from build123d import *

# Parameters (mm, degrees)
SKETCH_1_W                      = 158
SKETCH_1_H                      = 47.848101266
EXTRUDE_1_DEPTH                 = 2.5
CUT_EXTRUDE_1_REACH             = 84.581
SKETCH_2_W                      = 64
SKETCH_2_H                      = 27.924050633
CUT_EXTRUDE_2_REACH             = 84.581
SKETCH_4_R                      = 1.7
SKETCH_4_R_2                    = 1.8
CUT_EXTRUDE_3_REACH             = 84.581
SKETCH_5_R                      = 1.6
CUT_EXTRUDE_3_DIRECTION_2_DEPTH = 83.580931205
FILLET_4_R                      = 3
FILLET_5_R                      = 4
FILLET_6_R                      = 20
EXTRUDE_START                   = -79
EXTRUDE_2_DEPTH                 = 65
CUT_EXTRUDE_START               = -79
CUT_EXTRUDE_4_DEPTH             = 40
FILLET_7_R                      = 0.5
FILLET_8_R                      = 2
FILLET_9_R                      = 3
FILLET_10_R                     = 2
SKETCH_10_R                     = 1.6
CUT_EXTRUDE_5_DEPTH             = 95.325235224
SKETCH_11_R                     = 1.6
CUT_EXTRUDE_6_DEPTH             = 85.602511087


with BuildPart() as part:
    # 草图1 → 凸台-拉伸1 (new body)
    with BuildSketch(Plane(origin=(0, 0, 0), x_dir=(1, 0, 0), z_dir=(0, 1, 0))):
        Rectangle(SKETCH_1_W, SKETCH_1_H)
    extrude(amount=EXTRUDE_1_DEPTH)

    # 草图2 → 切除-拉伸1 (cut, up to next)
    with BuildSketch(Plane(origin=(0, 2.5, 0), x_dir=(1, 0, 0), z_dir=(0, 1, 0)), mode=Mode.PRIVATE) as cut_extrude_1_sk1:
        with Locations((-32, -9.962025317)):
            Rectangle(SKETCH_2_W, SKETCH_2_H)
    cut_extrude_1_tool1 = extrude(cut_extrude_1_sk1.sketch, amount=-CUT_EXTRUDE_1_REACH, mode=Mode.PRIVATE) & part.part
    # 草图2 → 切除-拉伸1 (cut, up to next)
    with BuildSketch(Plane(origin=(0, 2.5, 0), x_dir=(1, 0, 0), z_dir=(0, 1, 0)), mode=Mode.PRIVATE) as cut_extrude_1_sk2:
        with Locations((32, -9.962025317)):
            Rectangle(SKETCH_2_W, SKETCH_2_H)
    cut_extrude_1_tool2 = extrude(cut_extrude_1_sk2.sketch, amount=-CUT_EXTRUDE_1_REACH, mode=Mode.PRIVATE) & part.part
    add(cut_extrude_1_tool1.solids().sort_by_distance((-32, 2.5, 9.962025))[0], mode=Mode.SUBTRACT)
    add(cut_extrude_1_tool2.solids().sort_by_distance((32, 2.5, 9.962025))[0], mode=Mode.SUBTRACT)

    # 草图4 → 切除-拉伸2 (cut, up to next)
    with BuildSketch(Plane(origin=(0, 2.5, 0), x_dir=(1, 0, 0), z_dir=(0, 1, 0)), mode=Mode.PRIVATE) as cut_extrude_2_sk1:
        with Locations(Location((-74, -8.924050633, 0), (0, 0, 270))):
            Circle(SKETCH_4_R)
    cut_extrude_2_tool1 = extrude(cut_extrude_2_sk1.sketch, amount=-CUT_EXTRUDE_2_REACH, mode=Mode.PRIVATE) & part.part
    # 草图4 → 切除-拉伸2 (cut, up to next)
    with BuildSketch(Plane(origin=(0, 2.5, 0), x_dir=(1, 0, 0), z_dir=(0, 1, 0)), mode=Mode.PRIVATE) as cut_extrude_2_sk2:
        with Locations(Location((-74, 20.575949367, 0), (0, 0, 270))):
            Circle(SKETCH_4_R)
    cut_extrude_2_tool2 = extrude(cut_extrude_2_sk2.sketch, amount=-CUT_EXTRUDE_2_REACH, mode=Mode.PRIVATE) & part.part
    # 草图4 → 切除-拉伸2 (cut, up to next)
    with BuildSketch(Plane(origin=(0, 2.5, 0), x_dir=(1, 0, 0), z_dir=(0, 1, 0)), mode=Mode.PRIVATE) as cut_extrude_2_sk3:
        with Locations(Location((-74, -19.424050633, 0), (0, 0, 270))):
            Circle(SKETCH_4_R_2)
    cut_extrude_2_tool3 = extrude(cut_extrude_2_sk3.sketch, amount=-CUT_EXTRUDE_2_REACH, mode=Mode.PRIVATE) & part.part
    # 草图4 → 切除-拉伸2 (cut, up to next)
    with BuildSketch(Plane(origin=(0, 2.5, 0), x_dir=(1, 0, 0), z_dir=(0, 1, 0)), mode=Mode.PRIVATE) as cut_extrude_2_sk4:
        with Locations(Location((74, 20.575949367, 0), (0, 0, 270))):
            Circle(SKETCH_4_R)
    cut_extrude_2_tool4 = extrude(cut_extrude_2_sk4.sketch, amount=-CUT_EXTRUDE_2_REACH, mode=Mode.PRIVATE) & part.part
    # 草图4 → 切除-拉伸2 (cut, up to next)
    with BuildSketch(Plane(origin=(0, 2.5, 0), x_dir=(1, 0, 0), z_dir=(0, 1, 0)), mode=Mode.PRIVATE) as cut_extrude_2_sk5:
        with Locations(Location((74, -19.424050633, 0), (0, 0, 270))):
            Circle(SKETCH_4_R_2)
    cut_extrude_2_tool5 = extrude(cut_extrude_2_sk5.sketch, amount=-CUT_EXTRUDE_2_REACH, mode=Mode.PRIVATE) & part.part
    # 草图4 → 切除-拉伸2 (cut, up to next)
    with BuildSketch(Plane(origin=(0, 2.5, 0), x_dir=(1, 0, 0), z_dir=(0, 1, 0)), mode=Mode.PRIVATE) as cut_extrude_2_sk6:
        with Locations(Location((74, -8.924050633, 0), (0, 0, 270))):
            Circle(SKETCH_4_R)
    cut_extrude_2_tool6 = extrude(cut_extrude_2_sk6.sketch, amount=-CUT_EXTRUDE_2_REACH, mode=Mode.PRIVATE) & part.part
    add(cut_extrude_2_tool1.solids().sort_by_distance((-74, 2.5, 8.924051))[0], mode=Mode.SUBTRACT)
    add(cut_extrude_2_tool2.solids().sort_by_distance((-74, 2.5, -20.575949))[0], mode=Mode.SUBTRACT)
    add(cut_extrude_2_tool3.solids().sort_by_distance((-74, 2.5, 19.424051))[0], mode=Mode.SUBTRACT)
    add(cut_extrude_2_tool4.solids().sort_by_distance((74, 2.5, -20.575949))[0], mode=Mode.SUBTRACT)
    add(cut_extrude_2_tool5.solids().sort_by_distance((74, 2.5, 19.424051))[0], mode=Mode.SUBTRACT)
    add(cut_extrude_2_tool6.solids().sort_by_distance((74, 2.5, 8.924051))[0], mode=Mode.SUBTRACT)

    # 草图5 → 切除-拉伸3 (cut, up to next)
    with BuildSketch(Plane(origin=(0, 2.5, 0), x_dir=(1, 0, 0), z_dir=(0, 1, 0)), mode=Mode.PRIVATE) as cut_extrude_3_sk1:
        with Locations(Location((0, 14, 0), (0, 0, 90))):
            Circle(SKETCH_5_R)
    cut_extrude_3_tool1 = extrude(cut_extrude_3_sk1.sketch, amount=-CUT_EXTRUDE_3_REACH, mode=Mode.PRIVATE) & part.part
    # 草图5 → 切除-拉伸3 (cut, up to next)
    with BuildSketch(Plane(origin=(0, 2.5, 0), x_dir=(1, 0, 0), z_dir=(0, 1, 0)), mode=Mode.PRIVATE) as cut_extrude_3_sk2:
        with Locations(Location((-45, 14, 0), (0, 0, 90))):
            Circle(SKETCH_5_R)
    cut_extrude_3_tool2 = extrude(cut_extrude_3_sk2.sketch, amount=-CUT_EXTRUDE_3_REACH, mode=Mode.PRIVATE) & part.part
    # 草图5 → 切除-拉伸3 (cut, up to next)
    with BuildSketch(Plane(origin=(0, 2.5, 0), x_dir=(1, 0, 0), z_dir=(0, 1, 0)), mode=Mode.PRIVATE) as cut_extrude_3_sk3:
        with Locations(Location((45, 14, 0), (0, 0, 90))):
            Circle(SKETCH_5_R)
    cut_extrude_3_tool3 = extrude(cut_extrude_3_sk3.sketch, amount=-CUT_EXTRUDE_3_REACH, mode=Mode.PRIVATE) & part.part
    add(cut_extrude_3_tool1.solids().sort_by_distance((0, 2.5, -14))[0], mode=Mode.SUBTRACT)
    add(cut_extrude_3_tool2.solids().sort_by_distance((-45, 2.5, -14))[0], mode=Mode.SUBTRACT)
    add(cut_extrude_3_tool3.solids().sort_by_distance((45, 2.5, -14))[0], mode=Mode.SUBTRACT)

    # 草图5 → 切除-拉伸3 direction 2 (cut)
    with BuildSketch(Plane(origin=(0, 2.5, 0), x_dir=(1, 0, 0), z_dir=(0, 1, 0))):
        with Locations(Location((0, 14, 0), (0, 0, 90))):
            Circle(SKETCH_5_R)
        with Locations(Location((-45, 14, 0), (0, 0, 90))):
            Circle(SKETCH_5_R)
        with Locations(Location((45, 14, 0), (0, 0, 90))):
            Circle(SKETCH_5_R)
    extrude(amount=CUT_EXTRUDE_3_DIRECTION_2_DEPTH, mode=Mode.SUBTRACT)

    # 圆角4
    fillet_4_edges = [part.edges().sort_by_distance(p)[0] for p in [
        (79, 1.25, 23.924050633),
        (-79, 1.25, 23.924050633),
        (-79, 1.25, -23.924050633),
        (79, 1.25, -23.924050633),
    ]]
    fillet(fillet_4_edges, radius=FILLET_4_R)

    # 圆角5
    fillet_5_edges = [part.edges().sort_by_distance(p)[0] for p in [
        (64, 1.25, 23.924050633),
        (-64, 1.25, 23.924050633),
    ]]
    fillet(fillet_5_edges, radius=FILLET_5_R)

    # 圆角6
    fillet_6_edges = [part.edges().sort_by_distance(p)[0] for p in [
        (-64, 1.25, -4),
        (64, 1.25, -4),
    ]]
    fillet(fillet_6_edges, radius=FILLET_6_R)

    # 草图8 → 凸台-拉伸2 (add, symmetric)
    with BuildSketch(Plane.ZY.offset(79).offset(EXTRUDE_START)):
        Polygon((-22.743286719, 0), (-28.575949367, 0), (-28.575949367, 12.5), (-26.075949367, 12.5), (-26.075949367, 2.5), (-22.743286719, 2.5), align=None)
    extrude(amount=EXTRUDE_2_DEPTH, both=True)

    # 草图9 → 切除-拉伸4 (cut, symmetric)
    with BuildSketch(Plane.ZY.offset(79).offset(CUT_EXTRUDE_START)):
        Polygon((-28.575949367, 0), (-22.743286719, 0), (-22.743286719, 2.5), (-26.075949367, 2.5), (-26.075949367, 12.5), (-28.575949367, 12.5), align=None)
    extrude(amount=CUT_EXTRUDE_4_DEPTH, both=True, mode=Mode.SUBTRACT)

    # 圆角7
    fillet_7_edges = [part.edges().sort_by_distance(p)[0] for p in [
        (52.5, 2.5, -26.075949367),
        (-52.5, 2.5, -26.075949367),
    ]]
    fillet(fillet_7_edges, radius=FILLET_7_R)

    # 圆角8
    fillet_8_edges = [part.edges().sort_by_distance(p)[0] for p in [
        (52.5, 0, -28.575949367),
        (-52.5, 0, -28.575949367),
    ]]
    fillet(fillet_8_edges, radius=FILLET_8_R)

    # 圆角9
    fillet_9_edges = [part.edges().sort_by_distance(p)[0] for p in [
        (-65, 12.5, -27.325949367),
        (65, 12.5, -27.325949367),
        (40, 12.5, -27.325949367),
        (-40, 12.5, -27.325949367),
    ]]
    fillet(fillet_9_edges, radius=FILLET_9_R)

    # 圆角10
    fillet_10_edges = [part.edges().sort_by_distance(p)[0] for p in [
        (-65, 1.25, -23.924050633),
        (-40, 1.25, -22.743286719),
        (65, 1.25, -23.924050633),
        (40, 1.25, -22.743286719),
    ]]
    fillet(fillet_10_edges, radius=FILLET_10_R)

    # 草图10 → 切除-拉伸5 (cut, through all)
    with BuildSketch(Plane.XY.offset(-26.075949367)):
        with Locations((-57.5, 7.5)):
            Circle(SKETCH_10_R)
        with Locations((-47.5, 7.5)):
            Circle(SKETCH_10_R)
        with Locations(Location((47.5, 7.5, 0), (0, 0, 180))):
            Circle(SKETCH_10_R)
        with Locations(Location((57.5, 7.5, 0), (0, 0, 180))):
            Circle(SKETCH_10_R)
    extrude(amount=-CUT_EXTRUDE_5_DEPTH, mode=Mode.SUBTRACT)

    # 草图11 → 切除-拉伸6 (cut, through all)
    with BuildSketch(Plane(origin=(0, 2.5, 0), x_dir=(1, 0, 0), z_dir=(0, 1, 0))):
        with Locations(Location((-27, 14, 0), (0, 0, 270))):
            Circle(SKETCH_11_R)
        with Locations(Location((-21, 14, 0), (0, 0, 270))):
            Circle(SKETCH_11_R)
        with Locations(Location((21, 14, 0), (0, 0, 90))):
            Circle(SKETCH_11_R)
        with Locations(Location((27, 14, 0), (0, 0, 90))):
            Circle(SKETCH_11_R)
    extrude(amount=-CUT_EXTRUDE_6_DEPTH, mode=Mode.SUBTRACT)


solid = part.part
Verification items for the finished model (mm, model axes). A direction names the side the tool comes from. Coordinates: 2 decimals unless noted, no trailing zeros. Order: outer loops, then holes, each group sorted by start corner. A loop starts at its lowest first (then second) coordinate and runs counter-clockwise, first axis right, second up. Notation, with made-up numbers: M -17,82.5 L 7,82.5 A22 ccw 7,105.5 Z; hole C -31,46 d2. An arc over 180 degrees is marked long. One line per item, written item: value. Start each with the question number.
Item 1: Sectioned sample at A-A (x = 0). Enter the section's corners in (y, z), then the cut area to 3 significant figures.
Item 2: Sectioned sample at D-D (z = -8.5). Enter the section's corners in (x, y).
Item 3: Sectioned sample at C-C (x = -18). Enter the section's corners in (y, z), then the cut area to 3 significant figures.
Item 4: Sectioned sample at B-B (y = 11). Enter the section's corners in (x, z), then the cut area to 3 significant figures.
Item 5: Access from +Z, -Z, +X, -X, +Y, -Y to the whole of each face (thin tool, end or side, straight path). Record for faces 1 (the cylindrical face through (65.14, 1.23, 22.72)), 2 (the flat face through (65, 5, -27)), 3 (the flat face through (-1, 2.5, -7)).
Item 6: Mould release check, pull along Y, two halves, no side actions. Record for faces 4 (the cylindrical face through (64.14, 11.6, -27.31)), 5 (the cylindrical face through (-56.02, 6.89, -27.31)), 6 (the cylindrical face through (-19.92, 1.27, -15.18)): released by +Y, released by -Y, zero draft, split by the parting line, or undercut.
Item 7: Scan lines: probe 1 along Z at (x, y) = (-74, 1.3); probe 2 along Y at (x, z) = (-51, -23.5); probe 3 along Z at (x, y) = (-47, 4). Record each from-to range of solid material in increasing order.
Item 8: Gauge pin test, flat ends, axial feed: pin 1 (0.8 mm diameter, centred on y = 7, z = -27, fed in from -X); pin 2 (1.2 mm diameter, centred on x = -72.5, y = 1.5, fed in from -Z); pin 3 (2 mm diameter, centred on x = -16.5, y = 1.5, fed in from -Z). Record the tip position at first contact, or that the pin passes through.
Conclusion:
1. outline: M 0,-22.74 L 2.5,-22.74 L 2.5,-15.6 L 0,-15.6 Z; M 0,-12.4 L 2.5,-12.4 L 2.5,-4 L 0,-4 Z
1. area: 38.9 mm^2
2. outline: M -79,0 L 79,0 L 79,2.5 L -79,2.5 Z
3. outline: M 0,-22.74 L 2.5,-22.74 L 2.5,-4 L 0,-4 Z
3. area: 46.9 mm^2
4. outline: M -64.6,-28.58 L -40.4,-28.58 L -40.4,-26.08 L -64.6,-26.08 Z; M 40.4,-28.58 L 64.6,-28.58 L 64.6,-26.08 L 40.4,-26.08 Z
4. area: 121 mm^2
5. face 1: +Z, +Y, -Y
5. face 2: -Z, +X, +Y, -Y
5. face 3: +Z, +X, -X, +Y
6. face 4: released by +Y
6. face 5: undercut
6. face 6: zero draft
7. probe 1: z = -23.92 to -22.28, -18.88 to 7.22, 10.62 to 17.62, 21.22 to 23.92
7. probe 2: y = 0 to 2.5
7. probe 3: z = -28.58 to -26.08
8. pin 1: stops at x = -65
8. pin 2: stops at z = -23.92
8. pin 3: stops at z = -22.74
